Verification items for the finished model (mm, model axes). A direction names the side the tool comes from. Give positions to 0.01 mm unless a question says otherwise; leave off trailing zeros. Loops run counter-clockwise (first coordinate to the right, second up) from the corner with the lowest first, then second, coordinate; pieces in that order, holes last. Notation, with made-up numbers: (63.5, 53) -> (73.5, 53) arc R21 ccw to (73.5, 86) -> close; hole circle Ø11 at (18, 67.5). An arc over 180 degrees is marked (long way). Answer in a Markdown table with one row per item. Add a question column.
Q1. Material ranges on probe 1 along X at (y, z) = (-1, 24); probe 2 along Z at (x, y) = (-11, 12.5); probe 3 along X at (y, z) = (-8, 101.5), recorded low to high.
Q2. Set-up check for faces 1 (the face through (-14.985, 0.66, 80.922)), 2 (the face through (-9.02, -15.53, 0.37)): record each of +Z, -Z, +X, -X, +Y, -Y from which the full face is reachable in a straight line by a thin tool's end or side.
Q3. Section check A-A on z = 18.5. Enter the section's corners in (x, y).
Q4. Gauge pin test, flat ends, axial feed: P1, Ø4, axis at x = 9.5, y = 5.5, coming from the -Z side; P2, Ø5, axis at y = -5, z = 17.5, coming from the -X side; P3, Ø6, axis at y = -3, z = 75.5, coming from the +X side; P4, Ø1.5, axis at x = 1.5, z = 65, coming from the -Y side. Record the tip position at first contact, or that the pin passes through.
```python
from build123d import *

# Parameters (mm, degrees)
DODANIE_WYCI_GNI_CIE1_DEPTH = 5
SZKIC2_OUTSIDE_W            = 69.95
SZKIC2_OUTSIDE_H            = 64.592
SZKIC2_OUTSIDE_R            = 17.320508076
WYTNIJ_WYCI_GNI_CIE1_DEPTH  = 5
WYTNIJ_WYCI_GNI_CIE1_DRAFT  = 60
SZKIC3_R                    = 15
DODANIE_WYCI_GNI_CIE2_DEPTH = 155
SFAZOWANIE1_SIZE            = 1


with BuildPart() as part:
    # Szkic1 → Dodanie-wyciągnięcie1 (new body)
    with BuildSketch(Plane.XY):
        Polygon((10, 17.320508076), (-10, 17.320508076), (-20, 0), (-10, -17.320508076), (10, -17.320508076), (20, 0), align=None)
    extrude(amount=DODANIE_WYCI_GNI_CIE1_DEPTH)


with BuildPart() as wytnij_wyci_gni_cie1_tool:
    # Szkic2 outside → Wytnij-wyciągnięcie1 (with draft: the straight prism first)
    with BuildSketch(Plane.XY):
        Rectangle(SZKIC2_OUTSIDE_W, SZKIC2_OUTSIDE_H)
        Circle(SZKIC2_OUTSIDE_R, mode=Mode.SUBTRACT)
    extrude(amount=WYTNIJ_WYCI_GNI_CIE1_DEPTH)
    # Wytnij-wyciągnięcie1: the draft: its side faces are tilted about the plane it starts from
    wytnij_wyci_gni_cie1_sides = [wytnij_wyci_gni_cie1_tool.faces().sort_by_distance(p)[0] for p in [
        (0, -32.296, 2.5),
        (34.975, 0, 2.5),
        (0, 32.296, 2.5),
        (-34.975, 0, 2.5),
        (-17.320508076, 0, 2.5),
    ]]
    draft(wytnij_wyci_gni_cie1_sides, Plane.XY, WYTNIJ_WYCI_GNI_CIE1_DRAFT)


with BuildPart() as part_1:
    add(part.part)

    # Wytnij-wyciągnięcie1: cut by wytnij_wyci_gni_cie1_tool
    add(wytnij_wyci_gni_cie1_tool.part, mode=Mode.SUBTRACT)

    # Szkic3 → Dodanie-wyciągnięcie2 (add)
    with BuildSketch(Plane.XY.offset(5)):
        Circle(SZKIC3_R)
    extrude(amount=DODANIE_WYCI_GNI_CIE2_DEPTH)

    # Sfazowanie1
    sfazowanie1_edges = [part_1.edges().sort_by_distance(p)[0] for p in [
        (-15, 0, 160),
    ]]
    chamfer(sfazowanie1_edges, length=SFAZOWANIE1_SIZE)


solid = part_1.part
```
Taken from the geometry:
| question | item | result |
|---|---|---|
| 1 | probe 1 | x = -14.97 to 14.97 |
| 1 | probe 2 | z = 0 to 5 |
| 1 | probe 3 | x = -12.69 to 12.69 |
| 2 | face 1 | +Z |
| 2 | face 2 | -Z, -X, -Y |
| 3 | outline | circle Ø30 at (0, 0) |
| 4 | P1 | stops at z = 0 |
| 4 | P2 | stops at x = -14.79 |
| 4 | P3 | stops at x = 15 |
| 4 | P4 | stops at y = -14.98 |
